Check sheet for the drawn part. Datum: minimum x, y, z corner. Units: mm. A direction names the side the tool comes from. Give positions to 0.01 mm unless a question says otherwise; leave off trailing zeros. Order: outer loops, then holes, each group sorted by start corner. A loop starts at its lowest first (then second) coordinate and runs counter-clockwise, first axis right, second up.
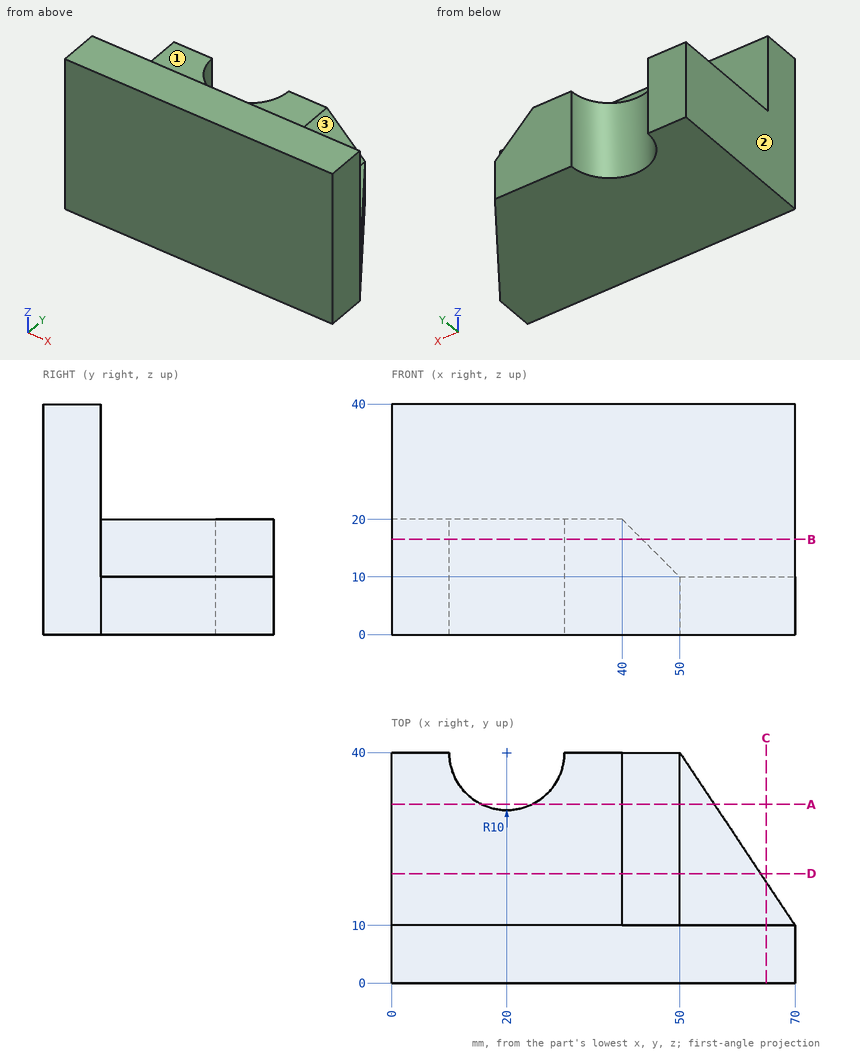
(1) Section check A-A, the plane y = 31. Enter the section's corners in (x, z), then the cut area to 3 significant figures.
Solved:
outline: (0, 0) - (15.64, 0) - (15.64, 20) - (0, 20) - close; (24.36, 0) - (56, 0) - (56, 10) - (50, 10) - (40, 20) - (24.36, 20) - close
area: 836 mm2
(2) Set-up check for the marked faces 1, 2 and 3: record each of +Z, -Z, +X, -X, +Y, -Y from which the full face is reachable in a straight line by a thin tool's end or side.
Solved:
face 1: +Z, +X, -X, +Y
face 2: +Z, -Z, -X, +Y, -Y
face 3: +Z, +X, +Y
(3) Section check D-D, the plane y = 19. Enter the section's corners in (x, z), then the cut area to 3 significant figures.
Solved:
outline: (0, 0) - (64, 0) - (64, 10) - (50, 10) - (40, 20) - (0, 20) - close
area: 1,090 mm2
(4) Scan lines: line 1 (Y direction, x = 56, z = 38.5); line 2 (X direction, y = 38, z = 12); line 3 (Z direction, x = 30, y = 25). Record each from-to range of solid material in increasing order.
Solved:
line 1: y = 0 to 10
line 2: x = 0 to 10.2, 29.8 to 48
line 3: z = 0 to 20
(5) Go/stop test with flat-tipped pins: pin 1 (2 mm diameter, centred on y = 11.5, z = 24.5, fed in from -X); pin 2 (3 mm diameter, centred on x = 16.5, y = 30, fed in from +Z); pin 3 (16 mm diameter, centred on x = 56, y = 24, fed in from +Z). Record where each tip stops, or that it passes through.
Solved:
pin 1: passes through
pin 2: stops at z = 20
pin 3: stops at z = 12
(6) Section check B-B, the plane z = 16.5. Enter the section's corners in (x, y), then the cut area to 3 significant figures.
Solved:
outline: (0, 0) - (70, 0) - (70, 10) - (43.5, 10) - (43.5, 40) - (30, 40) arc R10 cw to (10, 40) - (0, 40) - close
area: 1,850 mm2
(7) Section check C-C, the plane x = 65. Enter the section's corners in (y, z).
Solved:
outline: (0, 0) - (17.5, 0) - (17.5, 10) - (10, 10) - (10, 40) - (0, 40) - close
